Here's the drawing with two shaded views (mm, measured from the low corner). I have some questions. Coordinates: 2 decimals unless noted, no trailing zeros. Order: outer loops, then holes, each group sorted by start corner. A loop starts at its lowest first (then second) coordinate and runs counter-clockwise, first axis right, second up. Notation, with made-up numbers: (63.5, -9) - (102.5, -9) arc R29 ccw to (102.5, 18) - close; hole circle Ø10 at (84.5, 41.5). An arc over 180 degrees is marked (long way). One line per item, written item: value. Start each with the question number.
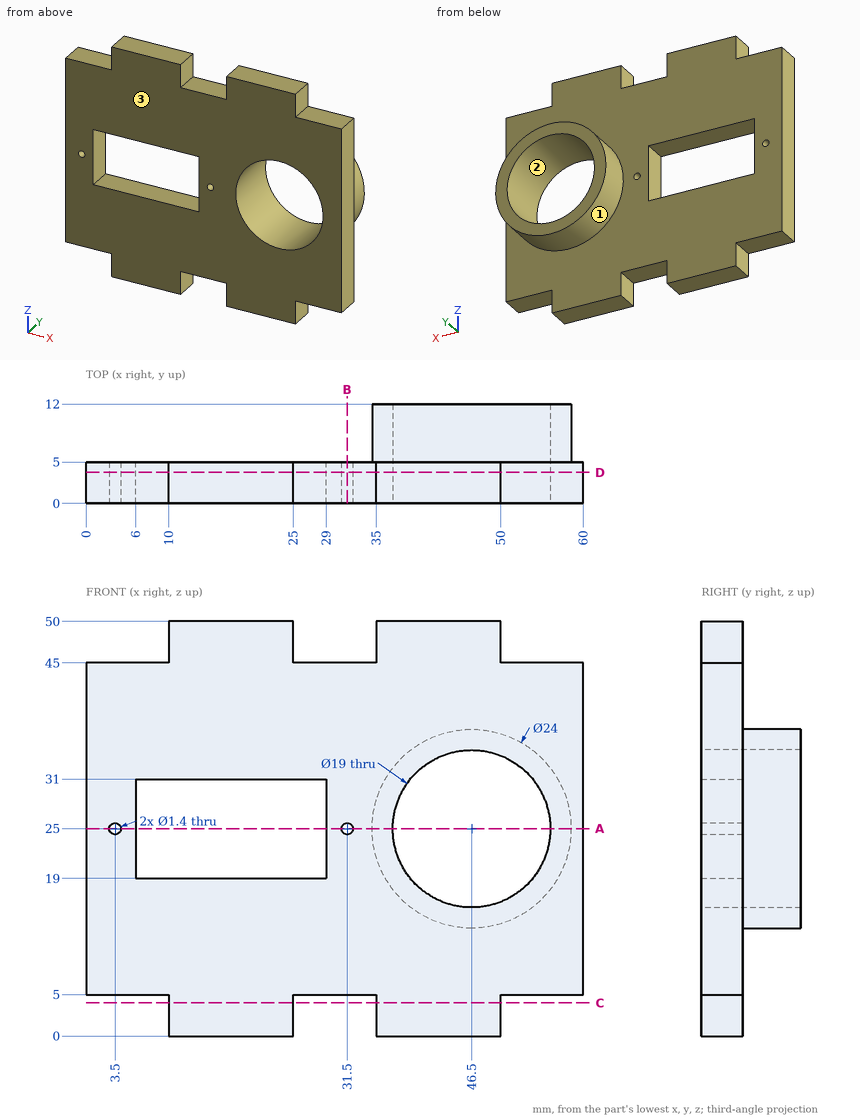
Q1. I want a section at C-C on z = 4. Please give me the cut outline in (x, y).
Q2. I want a section at A-A on z = 25. Please give me the cut outline in (x, y), then the cut area to 3 significant figures.
Q3. We'd pull the mould along X, two halves only. Please class the marked faces 1, 2 and 3: +X half, -X half, draft (parallel to the pull), parting line (faces both ways), or undercut.
Q4. I'm going to push flat-ended pins straight in: pin 1 (1.5 mm diameter, centred on y = 3.5, z = 47, fed in from -X); pin 2 (4 mm diameter, centred on x = 6.5, z = 25, fed in from +Y); pin 3 (1.5 mm diameter, centred on x = 5, y = 2.5, fed in from +Z). Where does each tip first touch, or does it pass through?
Q5. If I drill on L1, parallel to X at y = 2.75, z = 25; L2, parallel to Z at x = 9.5, y = 3; L3, parallel to Z at x = 11, y = 4.5, over which ranges is the centre line in solid material (lowest first)?
Q6. I want a section at D-D on y = 3.75. Please give me the cut outline in (x, z), then the cut area to 3 significant figures.
Q7. I want a section at B-B on x = 31.5. Please give me the cut outline in (y, z).
Values follow:
1. outline: (10, 0) - (25, 0) - (25, 5) - (10, 5) - close; (35, 0) - (50, 0) - (50, 5) - (35, 5) - close
2. outline: (0, 0) - (2.8, 0) - (2.8, 5) - (0, 5) - close; (4.2, 0) - (6, 0) - (6, 5) - (4.2, 5) - close; (29, 0) - (30.8, 0) - (30.8, 5) - (29, 5) - close; (32.2, 0) - (37, 0) - (37, 12) - (34.5, 12) - (34.5, 5) - (32.2, 5) - close; (56, 0) - (60, 0) - (60, 5) - (58.5, 5) - (58.5, 12) - (56, 12) - close
2. area: 111 mm^2
3. face 1: parting line
3. face 2: undercut
3. face 3: draft
4. pin 1: stops at x = 10
4. pin 2: stops at y = 5
4. pin 3: stops at z = 45
5. L1: x = 0 to 2.8, 4.2 to 6, 29 to 30.8, 32.2 to 37, 56 to 60
5. L2: z = 5 to 19, 31 to 45
5. L3: z = 0 to 19, 31 to 50
6. outline: (0, 5) - (10, 5) - (10, 0) - (25, 0) - (25, 5) - (35, 5) - (35, 0) - (50, 0) - (50, 5) - (60, 5) - (60, 45) - (50, 45) - (50, 50) - (35, 50) - (35, 45) - (25, 45) - (25, 50) - (10, 50) - (10, 45) - (0, 45) - close; hole circle Ø1.4 at (3.5, 25); hole (6, 19) - (29, 19) - (29, 31) - (6, 31) - close; hole circle Ø1.4 at (31.5, 25); hole circle Ø19 at (46.5, 25)
6. area: 2,140 mm^2
7. outline: (0, 5) - (5, 5) - (5, 24.3) - (0, 24.3) - close; (0, 25.7) - (5, 25.7) - (5, 45) - (0, 45) - close
